Part print with two shaded views. Sizes in mm from the minimum x, y, z corner. A direction names the side the tool comes from. Round coordinates to 2 decimals unless told otherwise and drop trailing zeros. Loops run counter-clockwise (first coordinate to the right, second up) from the corner with the lowest first, then second, coordinate; pieces in that order, holes last. Notation, with made-up numbers: M -28,8 L 31,8 A17 cw 31,33 Z; hole C 43,-28.5 d6. An arc over 180 degrees is marked long. Use a Markdown table: item, result. Add a question column.
Item 1: Tool access for the marked faces 1 and 2: list every direction of +Z, -Z, +X, -X, +Y, -Y with a clear straight run to the whole face (end or side of a thin tool).
Item 2: Pin check, flat tips, straight feed: P1, Ø6.5, axis at x = 4.5, z = 4.15, coming from the +Y side; P2, Ø1, axis at y = 16.5, z = 25.5, coming from the -X side; P3, Ø4, axis at x = 6, z = 20, coming from the -Y side. Stop position of each tip, or through.
Item 3: Wall check: L1, parallel to Z at x = 13.9, y = 13; L2, parallel to Z at x = 4.5, y = 19.9 (3 decimals); L3, parallel to X at y = 20.4, z = 4.15 (3 decimals). Give the ranges that are in metal, low to high. Write a range as from..to.
Item 4: Saw through at A-A on y = 13. Write the cut outline in (x, z), then the cut area to 4 significant figures.
Item 5: Saw through at C-C on x = 4.5. Write the cut outline in (y, z) (3 decimals).
Item 6: Saw through at D-D on y = 18.5. Write the cut outline in (x, z) (3 decimals).
Item 7: Saw through at B-B on z = 10.5. Write the cut outline in (x, y), then the cut area to 3 significant figures.
Item 8: Two-plate mould, pull along Z, no slides. Class the marked faces 3, 4 and 5: +Z half, -Z half, draft (parallel to the pull), parting line (faces both ways), or undercut.
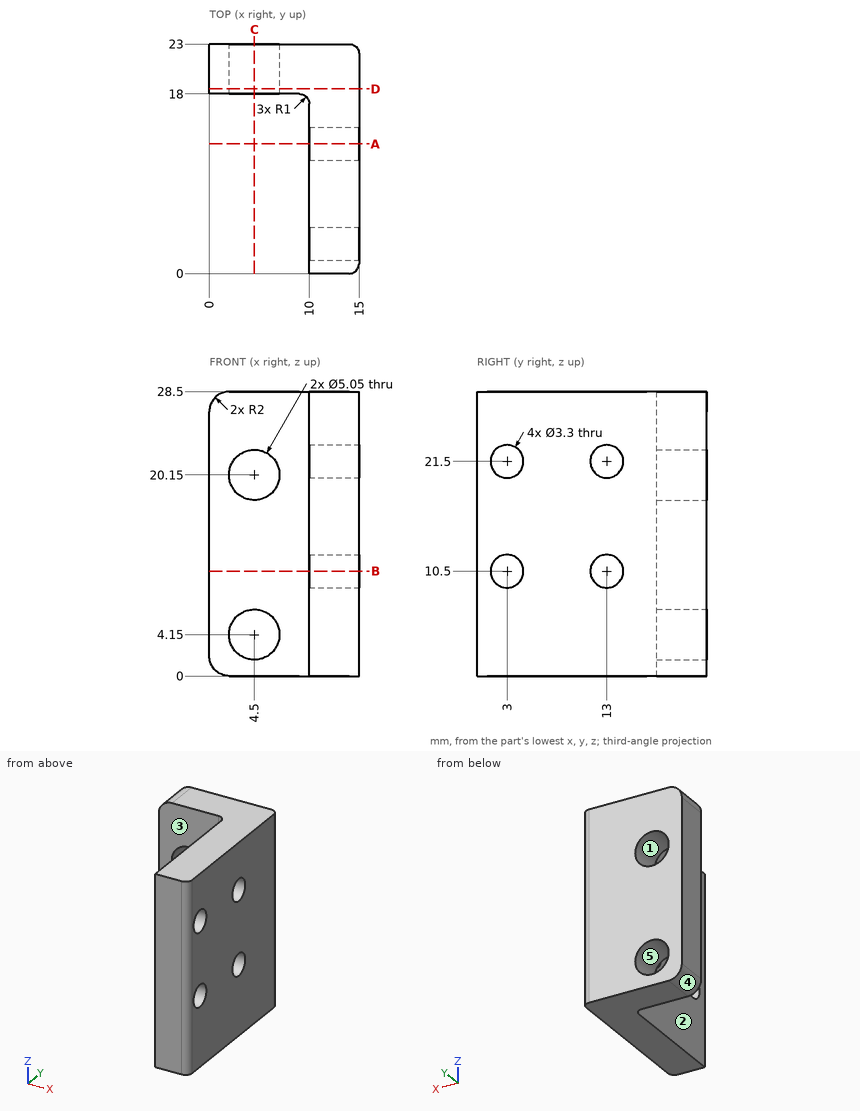
Entries:
| question | item | result |
|---|---|---|
| 1 | face 1 | +Y, -Y |
| 1 | face 2 | +Z, -Z, -X, -Y |
| 2 | P1 | y = 23 |
| 2 | P2 | x = 10 |
| 2 | P3 | y = 18 |
| 3 | L1 | 0..8.85, 12.15..19.85, 23.15..28.5 |
| 3 | L2 | 0..1.625, 6.675..17.625, 22.675..28.5 |
| 3 | L3 | 0..1.975, 7.025..15 |
| 4 | outline | M 10,0 L 15,0 L 15,8.85 L 10,8.85 Z; M 10,12.15 L 15,12.15 L 15,19.85 L 10,19.85 Z; M 10,23.15 L 15,23.15 L 15,28.5 L 10,28.5 Z |
| 4 | area | 109.5 mm2 |
| 5 | outline | M 18,0 L 23,0 L 23,1.625 L 18,1.625 Z; M 18,6.675 L 23,6.675 L 23,17.625 L 18,17.625 Z; M 18,22.675 L 23,22.675 L 23,28.5 L 18,28.5 Z |
| 6 | outline | M 0,2 A2 ccw 2,0 L 15,0 L 15,28.5 L 2,28.5 A2 ccw 0,26.5 Z; hole C 4.5,4.15 d5.05; hole C 4.5,20.15 d5.05 |
| 7 | outline | M 0,18 L 9,18 A1 cw 10,17 L 10,14.65 L 15,14.65 L 15,22 A1 ccw 14,23 L 0,23 Z; M 10,0 L 14,0 A1 ccw 15,1 L 15,1.35 L 10,1.35 Z; M 10,4.65 L 15,4.65 L 15,11.35 L 10,11.35 Z |
| 7 | area | 132 mm2 |
| 8 | face 3 | draft |
| 8 | face 4 | -Z half |
| 8 | face 5 | undercut |
